from build123d import *

# Parameters (mm, degrees)
F1_DEPTH = 30
F2_T     = -2.5
F3_R     = 5
F4_R     = 5


with BuildPart() as f1:
    # F0 (on Front) → F1 (new body)
    with BuildSketch(Plane.XZ):
        Polygon((-80.4619731335, 48.0414940363), (-80.4619731335, -90.2443051724), (80.4619731335, -90.2443051724), (80.4619731335, 48.0414940363), (32.4382460701, 72.9859998765), (32.4382460701, 140.1879998765), (-32.4382460701, 140.1879998765), (-32.4382460701, 72.9859998765), align=None)
    extrude(amount=F1_DEPTH)

    # F2
    f2_openings = [f1.faces().sort_by_distance(p)[0] for p in [
        (0, -30, 5.455809),
    ]]
    offset(amount=F2_T, openings=f2_openings, kind=Kind.INTERSECTION)

    # F3
    f3_edges = [f1.edges().sort_by_distance(p)[0] for p in [
        (-77.961973, -2.5, -20.610696),
        (-53.95011, -2.5, 58.995166),
        (-29.938246, -2.5, 104.577709),
        (0, -2.5, 137.688),
        (29.938246, -16.25, 137.688),
        (29.938246, -2.5, 104.577709),
        (53.95011, -2.5, 58.995166),
        (29.938246, -16.25, 71.467419),
        (-29.938246, -16.25, 71.467419),
        (-77.961973, -16.25, -87.744305),
        (0, -2.5, -87.744305),
        (77.961973, -16.25, -87.744305),
        (77.961973, -2.5, -20.610696),
        (-77.961973, -16.25, 46.522913),
        (-29.938246, -16.25, 137.688),
        (77.961973, -16.25, 46.522913),
    ]]
    fillet(f3_edges, radius=F3_R)

    # F4
    f4_edges = [f1.edges().sort_by_distance(p)[0] for p in [
        (32.438246, -15, 140.188),
        (80.461973, 0, -21.101406),
        (-32.438246, -15, 140.188),
        (-32.438246, -15, 72.986),
        (32.438246, -15, 72.986),
        (-80.461973, -15, 48.041494),
        (-80.461973, -15, -90.244305),
        (80.461973, -15, -90.244305),
    ]]
    fillet(f4_edges, radius=F4_R)


solid = f1.part
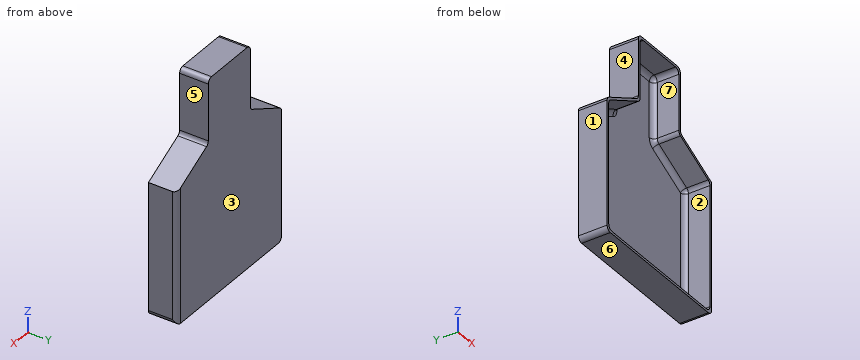
Geometry: final body of the model. Coordinates: model frame, mm. Face numbers are marked on the shaded views. A direction names the side the tool comes from. Round coordinates to 2 decimals unless told otherwise and drop trailing zeros. Loops run counter-clockwise (first coordinate to the right, second up) from the corner with the lowest first, then second, coordinate; pieces in that order, holes last.
Q1. Section D-D on z = 28. Return loops of the section in (x, y).
Q2. Pin query (flat end, axial travel): P1, Ø5, axis at x = 39, z = 60.5, coming from the -Y side; P2, Ø1, axis at x = 14.5, z = 29.5, coming from the -Y side; P3, Ø11, axis at y = -13.5, z = 110, coming from the +X side. Return the tip coordinate at first contact, or that it passes through.
Q3. Access query for the marked faces 4, 5, 6 and 7. Directions: +Z, -Z, +X, -X, +Y, -Y. A direction counts if a zero-diameter tool reaches every point of the face in a straight line with its end or side. Return the directions, or none.
Q4. Material intervals for L1, parallel to X at y = -22.5, z = 40; L2, parallel to X at y = -7.5, z = 104; L3, parallel to Y at x = 25, z = 60, sorted ascending.
Q5. Section B-B on z = 126. Return loops of the section in (x, y).
Q6. Section C-C on x = 6. Return loops of the section in (y, z).
Q7. Pull-direction query (X, two-part tool) for the marked faces 1, 2 and 3; classes: released by +X, released by -X, zero draft, split by the parting line, or undercut.
Evaluation:
1. outline: (-80.46, -30) - (-77.96, -30) - (-77.96, -7.5) arc R5 cw to (-72.96, -2.5) - (72.96, -2.5) arc R5 cw to (77.96, -7.5) - (77.96, -30) - (80.46, -30) - (80.46, -5) arc R5 ccw to (75.46, 0) - (-80.46, 0) - close
2. P1: stops at y = -2.89
2. P2: stops at y = -2.5
2. P3: stops at x = 32.44
3. face 4: +Z, -X, +Y, -Y
3. face 5: +Z, +X, +Y, -Y
3. face 6: -Z, +X, -X, +Y, -Y
3. face 7: -Y
4. L1: x = -80.46 to -77.96, 77.96 to 80.46
4. L2: x = -32.44 to -29.94, 29.94 to 32.44
4. L3: y = -2.5 to 0
5. outline: (-32.44, -30) - (-29.94, -30) - (-29.94, -7.5) arc R5 cw to (-24.94, -2.5) - (24.94, -2.5) arc R5 cw to (29.94, -7.5) - (29.94, -30) - (32.44, -30) - (32.44, 0) - (-32.44, 0) - close
6. outline: (-30, -90.24) - (0, -90.24) - (0, 140.19) - (-30, 140.19) - (-30, 137.69) - (-7.5, 137.69) arc R5 cw to (-2.5, 132.69) - (-2.5, -82.74) arc R5 cw to (-7.5, -87.74) - (-30, -87.74) - close
7. face 1: released by -X
7. face 2: undercut
7. face 3: zero draft
